```python
from build123d import *

# Parameters (mm, degrees)
BOSS_EXTRUDE1_DEPTH      = 20
BOSS_EXTRUDE1_DEPTH_BACK = 20
SKETCH1_R                = 3.5
BOSS_EXTRUDE2_DEPTH      = 10
BOSS_EXTRUDE3_START      = -10
BOSS_EXTRUDE3_DEPTH      = 10
CUT_EXTRUDE1_DEPTH       = 21
CUT_EXTRUDE1_DEPTH_BACK  = 22
SKETCH4_R                = 3.5
BOSS_EXTRUDE4_DEPTH      = 20
BOSS_EXTRUDE4_DEPTH_BACK = 20
SKETCH5_R                = 3.5
CUT_EXTRUDE2_DEPTH       = 23
CUT_EXTRUDE2_DEPTH_BACK  = 23
SKETCH6_R                = 3.5


with BuildPart() as part:
    # Sketch1 → Boss-Extrude1 (new, two sides: drawn at the far end of the back side and taken through both)
    with BuildSketch(Plane(origin=(0, 0, 0), x_dir=(1, 0, 0), z_dir=(0, 1, 0)).offset(-BOSS_EXTRUDE1_DEPTH_BACK)):
        with Locations(Location((-40, 0, 0), (0, 0, 270))):
            Circle(SKETCH1_R)
    extrude(amount=BOSS_EXTRUDE1_DEPTH + BOSS_EXTRUDE1_DEPTH_BACK)

    # Sketch2 → Boss-Extrude2 (add)
    with BuildSketch(Plane(origin=(0, 20, 0), x_dir=(1, 0, 0), z_dir=(0, 1, 0))):
        with BuildLine():
            Line((-40, 5), (0, 5))
            ThreePointArc((0, 5), (5, 0), (0, -5))
            Line((0, -5), (-40, -5))
            ThreePointArc((-40, -5), (-45, 0), (-40, 5))
        make_face()
    extrude(amount=-BOSS_EXTRUDE2_DEPTH)

    # Sketch3 → Boss-Extrude3 (add)
    with BuildSketch(Plane.XZ.offset(20).offset(BOSS_EXTRUDE3_START)):
        with BuildLine():
            Line((-40, 5), (0, 5))
            ThreePointArc((0, 5), (5, 0), (0, -5))
            Line((0, -5), (-40, -5))
            ThreePointArc((-40, -5), (-45, 0), (-40, 5))
        make_face()
    extrude(amount=BOSS_EXTRUDE3_DEPTH)

    # Sketch4 → Cut-Extrude1 (cut, two sides: drawn at the far end of the back side and taken through both)
    with BuildSketch(Plane(origin=(0, 0, 0), x_dir=(1, 0, 0), z_dir=(0, 1, 0)).offset(-CUT_EXTRUDE1_DEPTH_BACK)):
        with Locations(Location((0, 0, 0), (0, 0, 90))):
            Circle(SKETCH4_R)
    extrude(amount=CUT_EXTRUDE1_DEPTH + CUT_EXTRUDE1_DEPTH_BACK, mode=Mode.SUBTRACT)

    # Sketch5 → Boss-Extrude4 (add, two sides: drawn at the far end of the back side and taken through both)
    with BuildSketch(Plane(origin=(0, 0, 0), x_dir=(1, 0, 0), z_dir=(0, 1, 0)).offset(-BOSS_EXTRUDE4_DEPTH_BACK)):
        with Locations(Location((0, 0, 0), (0, 0, 270))):
            Circle(SKETCH5_R)
    extrude(amount=BOSS_EXTRUDE4_DEPTH + BOSS_EXTRUDE4_DEPTH_BACK)

    # Sketch6 → Cut-Extrude2 (cut, two sides: drawn at the far end of the back side and taken through both)
    with BuildSketch(Plane(origin=(0, 0, 0), x_dir=(1, 0, 0), z_dir=(0, 1, 0)).offset(-CUT_EXTRUDE2_DEPTH_BACK)):
        with Locations(Location((-40, 0, 0), (0, 0, 90))):
            Circle(SKETCH6_R)
    extrude(amount=CUT_EXTRUDE2_DEPTH + CUT_EXTRUDE2_DEPTH_BACK, mode=Mode.SUBTRACT)


solid = part.part
```
CAD build for the part. Positions are in the model's coordinates, mm. Give positions to 0.01 mm unless a question says otherwise; leave off trailing zeros. Loops run counter-clockwise (first coordinate to the right, second up) from the corner with the lowest first, then second, coordinate; pieces in that order, holes last. Notation, with made-up numbers: (70.25, 66) -> (86.25, 66) arc R5 cw to (86.25, 72) -> close; hole circle Ø2 at (12.25, 79). An arc over 180 degrees is marked (long way). Use a Markdown table: item, result.
1. Mould opens along Y. For faces 1 (the cylindrical face through (-3.417, -0.14, -0.759)), 2 (the flat face through (-20, -20, 0)), 3 (the flat face through (-20, 20, 0)), 4 (the cylindrical face through (-45, -15, 0)) say: pulls with the +Y half, pulls with the -Y half, needs draft (parallel to the pull), parting line crosses it, or undercut.
Check result:
| item | result |
|---|---|
| face 1 | undercut |
| face 2 | pulls with the -Y half |
| face 3 | pulls with the +Y half |
| face 4 | needs draft |
2. Wall check: L1, parallel to X at y = 17.25, z = 0; L2, parallel to Z at x = -40, y = 13; L3, parallel to Y at x = 0.5, z = 4.25. Give the ranges that are in metal, low to high. Write a range as [from, to].
Check result:
| item | result |
|---|---|
| L1 | x = [-45, -43.5], [-36.5, 5] |
| L2 | z = [-5, -3.5], [3.5, 5] |
| L3 | y = [-20, -10], [10, 20] |
3. Slice it at B-B (z = 0). List the corners of the cut face in (x, y).
Check result:
| item | result |
|---|---|
| outline | (-45, -20) -> (-43.5, -20) -> (-43.5, -10) -> (-45, -10) -> close; (-45, 10) -> (-43.5, 10) -> (-43.5, 20) -> (-45, 20) -> close; (-36.5, -20) -> (5, -20) -> (5, -10) -> (3.5, -10) -> (3.5, 10) -> (5, 10) -> (5, 20) -> (-36.5, 20) -> (-36.5, 10) -> (-3.5, 10) -> (-3.5, -10) -> (-36.5, -10) -> close |
4. Slice it at A-A (x = -5.5). List the corners of the cut face in (y, z), plus the area to 3 significant figures.
Check result:
| item | result |
|---|---|
| outline | (-20, -5) -> (-10, -5) -> (-10, 5) -> (-20, 5) -> close; (10, -5) -> (20, -5) -> (20, 5) -> (10, 5) -> close |
| area | 200 mm^2 |
5. Slice it at C-C (y = -16.5). List the corners of the cut face in (x, z).
Check result:
| item | result |
|---|---|
| outline | (-40, -5) -> (0, -5) arc R5 ccw to (0, 5) -> (-40, 5) arc R5 ccw to start; hole circle Ø7 at (-40, 0) |
6. Slice it at D-D (x = -41). List the corners of the cut face in (y, z), plus the area to 3 significant figures.
Check result:
| item | result |
|---|---|
| outline | (-20, -4.9) -> (-10, -4.9) -> (-10, -3.35) -> (-20, -3.35) -> close; (-20, 3.35) -> (-10, 3.35) -> (-10, 4.9) -> (-20, 4.9) -> close; (10, -4.9) -> (20, -4.9) -> (20, -3.35) -> (10, -3.35) -> close; (10, 3.35) -> (20, 3.35) -> (20, 4.9) -> (10, 4.9) -> close |
| area | 61.8 mm^2 |
7. Flat gauge pins, fed straight in: pin 1 (5.5 mm diameter, centred on x = -40, z = 0, fed in from -Y); pin 2 (1 mm diameter, centred on y = -0.5, z = -2.5, fed in from -X); pin 3 (6 mm diameter, centred on y = -1, z = -0.5, fed in from -X). Where does each tip first touch, or does it go through?
Check result:
| item | result |
|---|---|
| pin 1 | passes through |
| pin 2 | stops at x = -2.87 |
| pin 3 | stops at x = -3.5 |
